Source: CAD feature listing. Evaluate the final solid. Frame: model axes, mm. A direction names the side the tool comes from. Round coordinates to 2 decimals unless told otherwise and drop trailing zeros. Loops run counter-clockwise (first coordinate to the right, second up) from the corner with the lowest first, then second, coordinate; pieces in that order, holes last. Notation, with made-up numbers: M 89.25,88 L 117.25,88 A33 cw 117.25,123 Z; hole C 36,35.25 d11. An arc over 180 degrees is marked long. Answer as a JSON object with one key per item and string values.
from build123d import *

# Parameters (mm, degrees)
F0_R     = 1.65
F1_DEPTH = 3.5
F3_DEPTH = 6


with BuildPart() as f1:
    # F0 (on Top) → F1 (new body)
    with BuildSketch(Plane.XY):
        with BuildLine():
            Line((0, 6), (-71.800094, 6))
            ThreePointArc((-71.800094, 6), (-77.800094, 0), (-71.800094, -6))
            Line((-71.800094, -6), (0, -6))
            Line((0, -6), (11, -5))
            Line((11, -5), (83.678898, -5))
            ThreePointArc((83.678898, -5), (88.678898, 0), (83.678898, 5))
            Line((83.678898, 5), (11, 4.999999))
            Line((11, 4.999999), (0, 6))
        make_face()
        with Locations((46.678898, -0.051367)):
            Circle(F0_R, mode=Mode.SUBTRACT)
        with BuildLine():
            ThreePointArc((75.078858, 2.6), (77.678898, 1.9e-05), (75.078895, -2.6))
            Line((75.078895, -2.6), (55.290283, -2.599975))
            ThreePointArc((55.290283, -2.599975), (55.278895, -2.6), (55.267506, -2.599975))
            ThreePointArc((55.267506, -2.599975), (52.679025, 0.02565), (55.318805, 2.599694))
            Line((55.318805, 2.599694), (75.078858, 2.6))
        make_face(mode=Mode.SUBTRACT)
        with BuildLine():
            ThreePointArc((-71.800094, -2.6), (-74.400094, 0), (-71.800094, 2.6))
            Line((-71.800094, 2.6), (-47.000807, 2.6))
            ThreePointArc((-47.000807, 2.6), (-44.400807, 0), (-47.000807, -2.6))
            Line((-47.000807, -2.6), (-71.800094, -2.6))
        make_face(mode=Mode.SUBTRACT)
        with BuildLine():
            ThreePointArc((-30.8, -2.6), (-33.4, 0), (-30.8, 2.6))
            Line((-30.8, 2.6), (-6, 2.6))
            ThreePointArc((-6, 2.6), (-5.998491, 2.6), (-5.996982, 2.599998))
            ThreePointArc((-5.996982, 2.599998), (-3.400001, -0.001509), (-6, -2.6))
            Line((-6, -2.6), (-30.8, -2.6))
        make_face(mode=Mode.SUBTRACT)
        with Locations((83.678898, 0)):
            Circle(F0_R, mode=Mode.SUBTRACT)
    extrude(amount=F1_DEPTH)

    # F2 (on Front) → F3 (cut, symmetric)
    with BuildSketch(Plane.XZ):
        Polygon((-80.43514, 1), (-80.43514, 0), (11, 0), (0, 1), align=None)
    extrude(amount=F3_DEPTH, both=True, mode=Mode.SUBTRACT)


solid = f1.part
Item 1: Section A-A on z = 2.85. Give the number of separate pieces and of enclosed holes in the cut face, then the cut area to 3 significant figures.
Answer sheet:
{"separate pieces": "1", "enclosed holes": "5", "area": "1,360 mm²"}
Item 2: Contact query for flat-ended pins moving along their axis: pin 1 Ø3 at (x, y) = (83.68, 0) entering from -Z; pin 2 Ø1.8 at (x, z) = (67, 1) entering from +Y; pin 3 Ø1 at (x, z) = (48.5, 1.5) entering from -Y. Output: stop coordinate, or through.
Answer sheet:
{"pin 1": "passes through", "pin 2": "stops at y = 5", "pin 3": "stops at y = -5"}
Item 3: Pull-direction query (X, two-part tool) for faces 6 (the flat face through (-38, 0, 1)), 7 (the cylindrical face through (82.463, 1.115, 1.726)), 8 (the flat face through (5.577, -0.084, 0.493)), 9 (the cylindrical face through (45.03, 0.02, 1.73)); classes: pulls with the +X half, pulls with the -X half, needs draft (parallel to the pull), parting line crosses it, or undercut.
Answer sheet:
{"face 6": "needs draft", "face 7": "undercut", "face 8": "pulls with the -X half", "face 9": "undercut"}
Item 4: Access query for faces 1 (the cylindrical face through (-3.4, 0.1, 2.2)), 2 (the flat face through (48, 5, 2)), 3 (the cylindrical face through (-77.8, 0.1, 2.2)), 4 (the flat face through (47, -5, 2)), 5 (the cylindrical face through (88.678, -0.11, 1.726)). Directions: +Z, -Z, +X, -X, +Y, -Y. A direction counts if a zero-diameter tool reaches every point of the face in a straight line with its end or side. Return the directions, or none.
Answer sheet:
{"face 1": "+Z, -Z", "face 2": "+Z, -Z, +X, +Y", "face 3": "+Z, -Z, -X", "face 4": "+Z, -Z, +X, -Y", "face 5": "+Z, -Z, +X"}
Item 5: Line query: probe 1 along Y at (x, z) = (69, 1.9); probe 2 along Y at (x, z) = (-6, 1.2); probe 3 along Y at (x, z) = (21, 1.7). Output: solid intervals per line, ascending. Write a range as from..to.
Answer sheet:
{"probe 1": "y = -5..-2.6, 2.6..5", "probe 2": "y = -6..-2.6, 2.6..6", "probe 3": "y = -5..5"}
Item 6: Section B-B on x = 5.5. Return the cut outline in (y, z), then the cut area to 3 significant figures.
Answer sheet:
{"outline": "M -5.5,0.5 L 5.5,0.5 L 5.5,3.5 L -5.5,3.5 Z", "area": "33.0 mm²"}
